Work out the finished part from the listing and answer in its coordinate system (mm). Face numbers are marked on the shaded views. A direction names the side the tool comes from. Coordinates: 2 decimals unless noted, no trailing zeros. Order: outer loops, then holes, each group sorted by start corner. A loop starts at its lowest first (then second) coordinate and runs counter-clockwise, first axis right, second up.
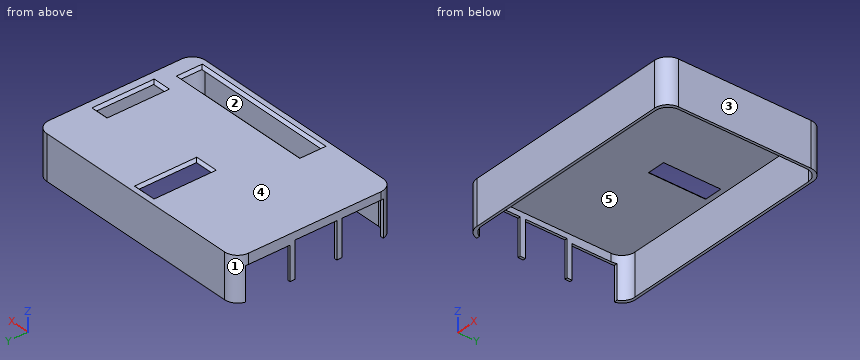
```python
from build123d import *

# Parameters (mm, degrees)
PAD_DEPTH       = 17
SKETCH001_W     = 55
SKETCH001_H     = 8
POCKET_DEPTH    = 17.001
CHAMFER_SIZE    = 1
SKETCH002_W     = 7
SKETCH002_H     = 22
POCKET001_DEPTH = 17.001
CHAMFER001_SIZE = 1
SKETCH003_W     = 5
SKETCH003_H     = 22
POCKET002_DEPTH = 17.001
CHAMFER002_SIZE = 1
POCKET003_DEPTH = 7
POCKET004_DEPTH = 16
SKETCH005_W     = 17
SKETCH005_H     = 13
SKETCH005_W_2   = 16
SKETCH005_H_2   = 14
POCKET005_DEPTH = 5


with BuildPart() as part:
    # Sketch → Pad (new body)
    with BuildSketch(Plane.XY):
        with BuildLine():
            Line((-41, 30.5), (41, 30.5))
            ThreePointArc((46, 25.5), (44.535534, 29.035534), (41, 30.5))
            Line((46, 25.5), (46, -25.5))
            ThreePointArc((41, -30.5), (44.535534, -29.035534), (46, -25.5))
            Line((41, -30.5), (-41, -30.5))
            ThreePointArc((-46, -25.5), (-44.535534, -29.035534), (-41, -30.5))
            Line((-46, -25.5), (-46, 25.5))
            ThreePointArc((-41, 30.5), (-44.535534, 29.035534), (-46, 25.5))
        make_face()
    extrude(amount=PAD_DEPTH)

    # Sketch001 (on Face10 of Pad) → Pocket (cut, through all)
    with BuildSketch(Plane.XY.offset(17)):
        with Locations((11.5, -23.5)):
            Rectangle(SKETCH001_W, SKETCH001_H)
    extrude(amount=-POCKET_DEPTH, mode=Mode.SUBTRACT)

    # Chamfer
    chamfer_edges = [part.edges().sort_by_distance(p)[0] for p in [
        (11.5, -27.5, 17),
        (-16, -23.5, 17),
        (11.5, -19.5, 17),
        (39, -23.5, 17),
    ]]
    chamfer(chamfer_edges, length=CHAMFER_SIZE)

    # Sketch002 (on Face1 of Chamfer) → Pocket001 (cut, through all)
    with BuildSketch(Plane.XY.offset(17)):
        with Locations((-1.5, 16.5)):
            Rectangle(SKETCH002_W, SKETCH002_H)
    extrude(amount=-POCKET001_DEPTH, mode=Mode.SUBTRACT)

    # Chamfer001
    chamfer001_edges = [part.edges().sort_by_distance(p)[0] for p in [
        (-5, 16.5, 17),
        (-1.5, 27.5, 17),
        (2, 16.5, 17),
        (-1.5, 5.5, 17),
    ]]
    chamfer(chamfer001_edges, length=CHAMFER001_SIZE)

    # Sketch003 (on Face1 of Chamfer001) → Pocket002 (cut, through all)
    with BuildSketch(Plane.XY.offset(17)):
        with Locations((39.5, -0.5)):
            Rectangle(SKETCH003_W, SKETCH003_H)
    extrude(amount=-POCKET002_DEPTH, mode=Mode.SUBTRACT)

    # Chamfer002
    chamfer002_edges = [part.edges().sort_by_distance(p)[0] for p in [
        (39.5, -11.5, 17),
        (42, -0.5, 17),
        (37, -0.5, 17),
        (39.5, 10.5, 17),
    ]]
    chamfer(chamfer002_edges, length=CHAMFER002_SIZE)

    # Sketch004 (on Face26 of Chamfer002) → Pocket003 (cut)
    with BuildSketch(Plane(origin=(0, 0, 0), x_dir=(1, 0, 0), z_dir=(0, 0, -1))):
        with BuildLine():
            Line((-40, 29.5), (40, 29.5))
            ThreePointArc((45, 24.5), (43.535534, 28.035534), (40, 29.5))
            Line((45, 24.5), (45, -24.5))
            ThreePointArc((40, -29.5), (43.535534, -28.035534), (45, -24.5))
            Line((40, -29.5), (-40, -29.5))
            ThreePointArc((-45, -24.5), (-43.535534, -28.035534), (-40, -29.5))
            Line((-45, -24.5), (-45, 24.5))
            ThreePointArc((-40, 29.5), (-43.535534, 28.035534), (-45, 24.5))
        make_face()
    extrude(amount=-POCKET003_DEPTH, mode=Mode.SUBTRACT)

    # Sketch004 (on Face26 of Chamfer002) → Pocket004 (cut)
    with BuildSketch(Plane(origin=(0, 0, 0), x_dir=(1, 0, 0), z_dir=(0, 0, -1))):
        with BuildLine():
            Line((-40, 29.5), (40, 29.5))
            ThreePointArc((45, 24.5), (43.535534, 28.035534), (40, 29.5))
            Line((45, 24.5), (45, -24.5))
            ThreePointArc((40, -29.5), (43.535534, -28.035534), (45, -24.5))
            Line((40, -29.5), (-40, -29.5))
            ThreePointArc((-45, -24.5), (-43.535534, -28.035534), (-40, -29.5))
            Line((-45, -24.5), (-45, 24.5))
            ThreePointArc((-40, 29.5), (-43.535534, 28.035534), (-45, 24.5))
        make_face()
    extrude(amount=-POCKET004_DEPTH, mode=Mode.SUBTRACT)

    # Sketch005 (on Face6 of Pocket004) → Pocket005 (cut)
    with BuildSketch(Plane(origin=(-46, 0, 0), x_dir=(0, -1, 0), z_dir=(-1, 0, 0))):
        with Locations((-18, 6.5)):
            Rectangle(SKETCH005_W, SKETCH005_H)
        with Locations((0.5, 7)):
            Rectangle(SKETCH005_W_2, SKETCH005_H_2)
        with Locations((18.5, 7)):
            Rectangle(SKETCH005_W_2, SKETCH005_H_2)
    extrude(amount=-POCKET005_DEPTH, mode=Mode.SUBTRACT)


solid = part.part
```
1. For the marked faces 1 and 2, determine the directions among +Z, -Z, +X, -X, +Y, -Y from which every point of the face is accessible in a straight line to the end or side of a thin tool.
2. The part is cut by section D-D (x = 22). Determine the outline of the cut face in (y, z), plus the area to 3 significant figures.
3. The mould has two halves that part along X. Classify the marked faces 3, 4 and 5: released by +X, released by -X, zero draft, split by the parting line, or undercut.
4. The part is cut by section B-B (x = -3). Determine the outline of the cut face in (y, z), plus the area to 3 significant figures.
5. Flat-ended cylindrical pins translate along their axes: pin 1 (4 mm diameter, centred on x = 1.5, y = 13.5, fed in from -Z); pin 2 (1.1 mm diameter, centred on x = -45, z = 9, fed in from -Y); pin 3 (0.5 mm diameter, centred on x = -45.5, z = 8.5, fed in from +Y). Find the tip coordinate at first contact, or state that the pin passes through.
6. The part is cut by section A-A (y = -23.5). Determine the outline of the cut face in (x, z).
7. Consider probe 1 along Y at (x, z) = (21, 10.75); probe 2 along X at (y, z) = (-17.5, 14.25); probe 3 along Z at (x, y) = (32, -14). Determine where each line is inside the solid, lowest interval first.
8. The part is cut by section C-C (z = 3.25). Determine the outline of the cut face in (x, y).
Worked out:
1. face 1: +Z, -Z, -X, +Y
1. face 2: -Z
2. outline: (-30.5, 0) - (-29.5, 0) - (-29.5, 16) - (-27.5, 16) - (-28.5, 17) - (-30.5, 17) - close; (-19.5, 16) - (29.5, 16) - (29.5, 0) - (30.5, 0) - (30.5, 17) - (-18.5, 17) - close
2. area: 84.0 mm2
3. face 3: released by +X
3. face 4: zero draft
3. face 5: undercut
4. outline: (-30.5, 0) - (-29.5, 0) - (-29.5, 16) - (-27.5, 16) - (-28.5, 17) - (-30.5, 17) - close; (-19.5, 16) - (5.5, 16) - (4.5, 17) - (-18.5, 17) - close; (27.5, 16) - (29.5, 16) - (29.5, 0) - (30.5, 0) - (30.5, 17) - (28.5, 17) - close
4. area: 61.0 mm2
5. pin 1: stops at z = 16
5. pin 2: stops at y = -29.12
5. pin 3: stops at y = 28.13
6. outline: (-46, 14) - (-45, 14) - (-45, 16) - (-16, 16) - (-17, 17) - (-46, 17) - close; (39, 16) - (45, 16) - (45, 0) - (46, 0) - (46, 17) - (40, 17) - close
7. probe 1: y = -30.5 to -29.5, 29.5 to 30.5
7. probe 2: x = -46 to -45, 45 to 46
7. probe 3: z = 16 to 17
8. outline: (-46, -10.5) - (-45, -10.5) - (-45, -8.5) - (-46, -8.5) - close; (-46, 7.5) - (-45, 7.5) - (-45, 9.5) - (-46, 9.5) - close; (-45.9, -26.5) arc R5 ccw to (-41, -30.5) - (41, -30.5) arc R5 ccw to (46, -25.5) - (46, 25.5) arc R5 ccw to (41, 30.5) - (-41, 30.5) arc R5 ccw to (-45.9, 26.5) - (-44.58, 26.5) arc R5 cw to (-40, 29.5) - (40, 29.5) arc R5 cw to (45, 24.5) - (45, -24.5) arc R5 cw to (40, -29.5) - (-40, -29.5) arc R5 cw to (-44.58, -26.5) - close
